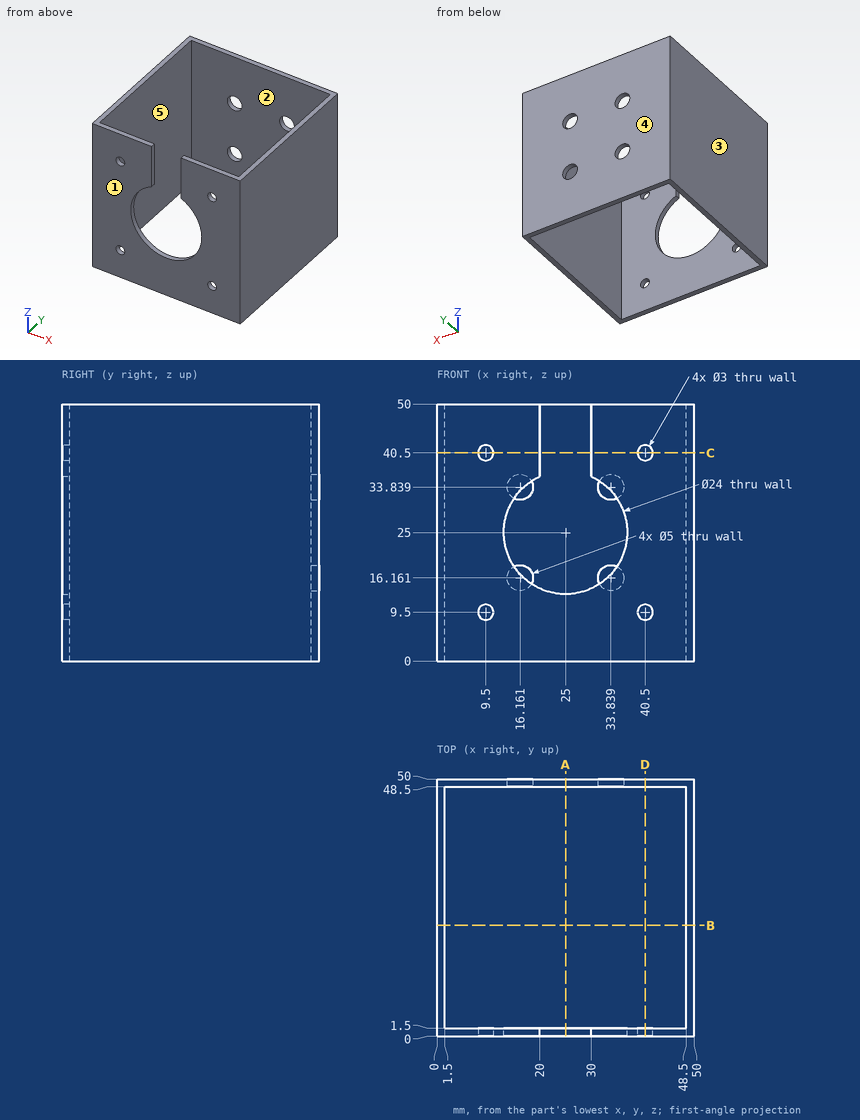
Drawing for the job (mm, zero at the part's lowest x, y, z). A direction names the side the tool comes from. Round coordinates to 2 decimals unless told otherwise and drop trailing zeros. Write each loop counter-clockwise with the first axis right and the second up, starting at its lowest first coordinate (ties: lowest second). Pieces come first, ordered by that corner, then holes. Notation, with made-up numbers: M 66,60.5 L 121,60.5 A15 cw 121,83.5 Z; hole C 75.5,5.5 d2. An arc over 180 degrees is marked long. Answer as a JSON object with one key per item and string values. Group by question number.
(1) Cut at C-C (z = 40.5). Give the cut face in (x, y), and give its area (3 significant figures).
(2) Which spindle directions (+Z, -Z, +X, -X, +Y, -Y) get a long thin tool onto all of the face, cutting with end or side? Do the marked faces 1 and 2. Say none if no direction does.
(3) Cut at A-A (x = 25). Give the cut face in (y, z), and give its area (3 significant figures).
(4) Cut at D-D (x = 40.5). Give the cut face in (y, z), and give its area (3 significant figures).
(5) Cut at B-B (y = 21.5). Give the cut face in (x, z).
(6) Mould opens along Y. For the marked faces 3, 4 and 5 say: pulls with the +Y half, pulls with the -Y half, needs draft (parallel to the pull), parting line crosses it, or undercut.
(7) Drill centre lines: L1, parallel to Z at x = 40.5, y = 0.65; L2, parallel to X at y = 30, z = 48. Where is each one in solid material? Low to high.
(8) Flat gauge pins, fed straight in: pin 1 (4.5 mm diameter, centred on x = 33.84, z = 16.16, fed in from +Y); pin 2 (5 mm diameter, centred on x = 30.5, z = 26, fed in from -Y); pin 3 (8 mm diameter, centred on x = 33.5, z = 21.5, fed in from -Y). Where does each tip first touch, or does it go through?
Responses:
{
 "1": {"outline": "M 0,0 L 8,0 L 8,1.5 L 1.5,1.5 L 1.5,48.5 L 48.5,48.5 L 48.5,1.5 L 42,1.5 L 42,0 L 50,0 L 50,50 L 0,50 Z; M 11,0 L 20,0 L 20,1.5 L 11,1.5 Z; M 30,0 L 39,0 L 39,1.5 L 30,1.5 Z", "area": "267 mm2"},
 "2": {"face 1": "+Z, -Z, +X, -X, -Y", "face 2": "+Z, -Z"},
 "3": {"outline": "M 0,0 L 1.5,0 L 1.5,13 L 0,13 Z; M 48.5,0 L 50,0 L 50,50 L 48.5,50 Z", "area": "94.5 mm2"},
 "4": {"outline": "M 0,0 L 1.5,0 L 1.5,8 L 0,8 Z; M 0,11 L 1.5,11 L 1.5,39 L 0,39 Z; M 0,42 L 1.5,42 L 1.5,50 L 0,50 Z; M 48.5,0 L 50,0 L 50,50 L 48.5,50 Z", "area": "141 mm2"},
 "5": {"outline": "M 0,0 L 1.5,0 L 1.5,50 L 0,50 Z; M 48.5,0 L 50,0 L 50,50 L 48.5,50 Z"},
 "6": {"face 3": "needs draft", "face 4": "pulls with the +Y half", "face 5": "undercut"},
 "7": {"L1": "z = 0 to 8, 11 to 39, 42 to 50", "L2": "x = 0 to 1.5, 48.5 to 50"},
 "8": {"pin 1": "stops at y = 1.5", "pin 2": "stops at y = 48.5", "pin 3": "stops at y = 0"}
}
